Can you work these out from the drawing? Everything is in mm from the part's minimum corner. A direction names the side the tool comes from. Round coordinates to 2 decimals unless told otherwise and drop trailing zeros. Write each loop counter-clockwise with the first axis right and the second up, starting at its lowest first coordinate (ties: lowest second). Pieces come first, ordered by that corner, then holes. Notation, with made-up numbers: (32.5, 48.25) -> (45.5, 48.25) arc R11 cw to (45.5, 62.25) -> close; hole circle Ø9 at (68, 10). An arc over 180 degrees is marked (long way). Write item = value, one per line. Start each with the question number.
1) If I drill on line 1 (Z direction, x = 79, y = 39); line 2 (X direction, y = 48, z = 67) (1 decimal); line 3 (X direction, y = 37.25, z = 115), over which ranges is the centre line in solid material (lowest first)?
2) Imagine slicing it at C-C, the plane z = 283. Please give me the cut outline in (x, y), then the cut area to 3 significant figures.
3) For the marked faces 4 and 5, which set-ups out of +Z, -Z, +X, -X, +Y, -Y let a thin tool reach every point of the face, with its end or its side?
4) I'm going to push flat-ended pins straight in: pin 1 (12 mm diameter, centred on y = 16.5, z = 261.5, fed in from -X); pin 2 (4 mm diameter, centred on x = 261, z = 132, fed in from +Y). Where does each tip first touch, or does it pass through?
5) Imagine slicing it at A-A, the plane x = 81. Please give me the cut outline in (y, z).
6) Thinking about a two-plate mould opening in X: for the marked faces 1, 2 and 3, which applies, +X half, -X half, draft (parallel to the pull), parting line (faces both ways), or undercut?
7) Imagine slicing it at B-B, the plane y = 51. Please give me the cut outline in (x, z).
8) Imagine slicing it at D-D, the plane x = 212. Please give me the cut outline in (y, z), then the cut area to 3 significant figures.
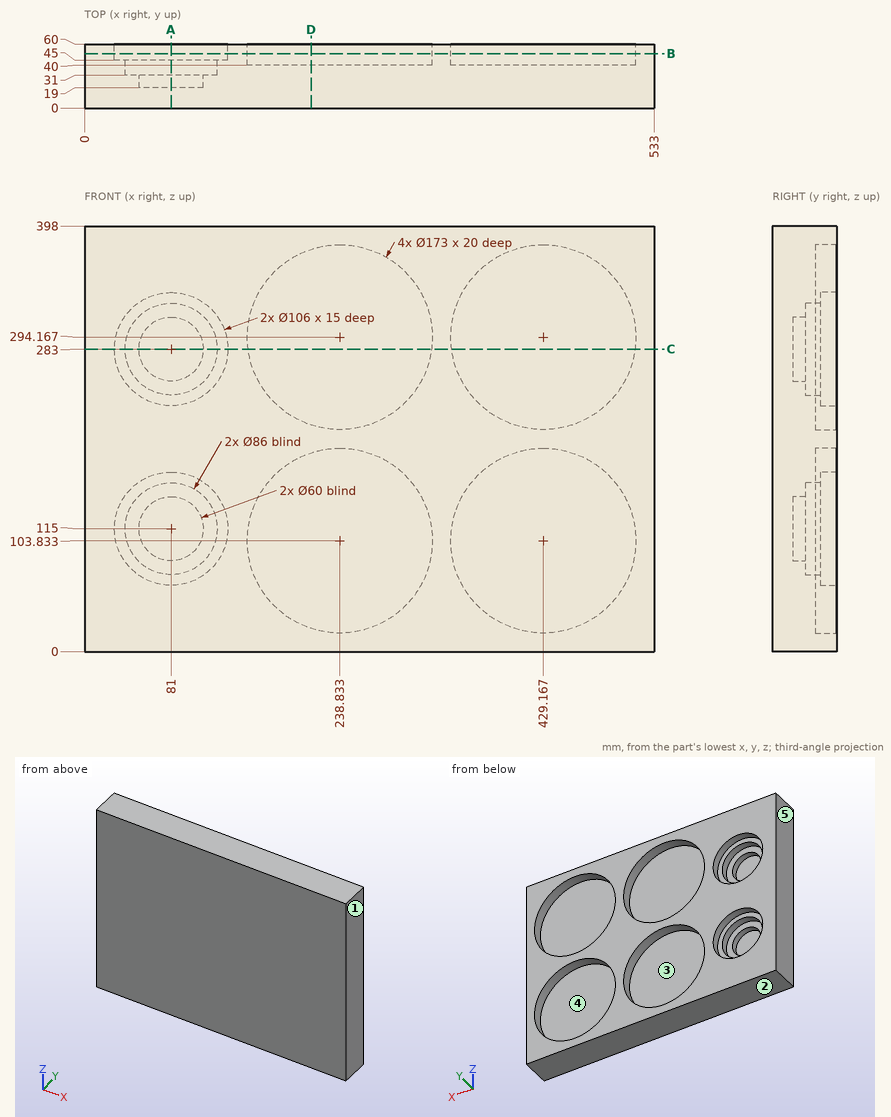
Reported:
q1.line_1 = 0 to 72.05, 157.95 to 240.05, 325.95 to 398
q1.line_2 = 0 to 58.5, 103.5 to 160.6, 317.1 to 350.9, 507.4 to 533
q1.line_3 = 0 to 38, 124 to 533
q2.outline = (0, 0) -> (533, 0) -> (533, 60) -> (514.94, 60) -> (514.94, 40) -> (343.39, 40) -> (343.39, 60) -> (324.61, 60) -> (324.61, 40) -> (153.06, 40) -> (153.06, 60) -> (134, 60) -> (134, 45) -> (124, 45) -> (124, 31) -> (111, 31) -> (111, 19) -> (51, 19) -> (51, 31) -> (38, 31) -> (38, 45) -> (28, 45) -> (28, 60) -> (0, 60) -> close
q2.area = 21,600 mm²
q3.face_4 = +Y
q3.face_5 = +Z, -Z, -X, +Y, -Y
q4.pin_1 = 0
q4.pin_2 = 40
q5.outline = (0, 0) -> (60, 0) -> (60, 62) -> (45, 62) -> (45, 72) -> (31, 72) -> (31, 85) -> (19, 85) -> (19, 145) -> (31, 145) -> (31, 158) -> (45, 158) -> (45, 168) -> (60, 168) -> (60, 230) -> (45, 230) -> (45, 240) -> (31, 240) -> (31, 253) -> (19, 253) -> (19, 313) -> (31, 313) -> (31, 326) -> (45, 326) -> (45, 336) -> (60, 336) -> (60, 398) -> (0, 398) -> close
q6.face_1 = +X half
q6.face_2 = draft
q6.face_3 = undercut
q7.outline = (0, 0) -> (533, 0) -> (533, 398) -> (0, 398) -> close; hole circle Ø106 at (81, 115); hole circle Ø106 at (81, 283); hole circle Ø173 at (238.83, 103.83); hole circle Ø173 at (238.83, 294.17); hole circle Ø173 at (429.17, 103.83); hole circle Ø173 at (429.17, 294.17)
q8.outline = (0, 0) -> (60, 0) -> (60, 21.6) -> (40, 21.6) -> (40, 186.07) -> (60, 186.07) -> (60, 211.93) -> (40, 211.93) -> (40, 376.4) -> (60, 376.4) -> (60, 398) -> (0, 398) -> close
q8.area = 17,300 mm²
